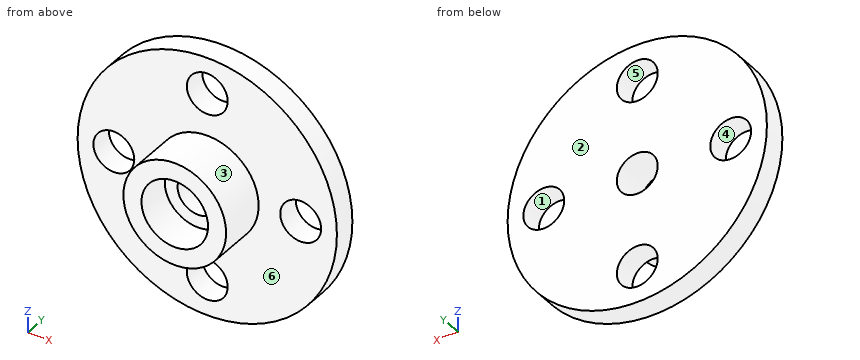
```python
from build123d import *

# Parameters (mm, degrees)
SKETCH1_R          = 11.1
EXTRUDE1_DEPTH     = 2
SKETCH2_R          = 1.75
CUT_EXTRUDE1_DEPTH = 3
SKETCH3_R          = 4.4
EXTRUDE2_DEPTH     = 4.2
SKETCH4_R          = 2.85
CUT_EXTRUDE2_DEPTH = 3
SKETCH5_R          = 1.75
CUT_EXTRUDE3_DEPTH = 4.2


with BuildPart() as part:
    # Sketch1 → Extrude1 (new body)
    with BuildSketch(Plane(origin=(0, 0, 0), x_dir=(1, 0, 0), z_dir=(0, 1, 0))):
        Circle(SKETCH1_R)
    extrude(amount=EXTRUDE1_DEPTH)

    # Sketch2 → Cut-Extrude1 (cut, through all)
    with BuildSketch(Plane(origin=(0, 2, 0), x_dir=(1, 0, 0), z_dir=(0, 1, 0))):
        with Locations((0, 8)):
            Circle(SKETCH2_R)
        with Locations((8, 0)):
            Circle(SKETCH2_R)
        with Locations((0, -8)):
            Circle(SKETCH2_R)
        with Locations((-8, 0)):
            Circle(SKETCH2_R)
    extrude(amount=-CUT_EXTRUDE1_DEPTH, mode=Mode.SUBTRACT)

    # Sketch3 → Extrude2 (add)
    with BuildSketch(Plane.XZ):
        Circle(SKETCH3_R)
    extrude(amount=EXTRUDE2_DEPTH)

    # Sketch4 → Cut-Extrude2 (cut)
    with BuildSketch(Plane.XZ.offset(4.2)):
        Circle(SKETCH4_R)
    extrude(amount=-CUT_EXTRUDE2_DEPTH, mode=Mode.SUBTRACT)

    # Sketch5 → Cut-Extrude3 (cut, through all)
    with BuildSketch(Plane.XZ.offset(1.2)):
        Circle(SKETCH5_R)
    extrude(amount=-CUT_EXTRUDE3_DEPTH, mode=Mode.SUBTRACT)


solid = part.part
```
Can you work these out from the model? Positions are in its coordinate system, mm. Face numbers are marked on the shaded views. A direction names the side the tool comes from. Coordinates: 2 decimals unless noted, no trailing zeros. Order: outer loops, then holes, each group sorted by start corner. A loop starts at its lowest first (then second) coordinate and runs counter-clockwise, first axis right, second up.
1. For the marked faces 5 and 6, which set-ups out of +Z, -Z, +X, -X, +Y, -Y let a thin tool reach every point of the face, with its end or its side?
2. If we section it at A-A (z = 0): Please give me the cut outline in (x, y).
3. If we section it at D-D (y = 0.5): Please give me the cut outline in (x, z).
4. Thinking about a two-plate mould opening in Z: for the marked faces 1, 2, 3 and 4, which applies, +Z half, -Z half, draft (parallel to the pull), parting line (faces both ways), or undercut?
5. If we section it at C-C (x = -8): Please give me the cut outline in (y, z), then the cut area to 3 significant figures.
6. If we section it at B-B (x = 0): Please give me the cut outline in (y, z), then the cut area to 3 significant figures.
7. I'm going to push a flat-ended pin straight in: pin 1 (4 mm diameter, centred on x = 0, z = 8, fed in from -Y). Where does the tip first touch, or does it pass through?
8. I need wall thicknesses on line 1 (Z direction, x = 0, y = 0.5); line 2 (Z direction, x = 0, y = -2.25); line 3 (X direction, y = 1.25, z = 8.25). Which ranges of each line are inside material? Lowest first, please.
Entries:
1. face 5: +Y, -Y
1. face 6: -Y
2. outline: (-11.1, 0) - (-9.75, 0) - (-9.75, 2) - (-11.1, 2) - close; (-6.25, 0) - (-4.4, 0) - (-4.4, -4.2) - (-2.85, -4.2) - (-2.85, -1.2) - (-1.75, -1.2) - (-1.75, 2) - (-6.25, 2) - close; (1.75, -1.2) - (2.85, -1.2) - (2.85, -4.2) - (4.4, -4.2) - (4.4, 0) - (6.25, 0) - (6.25, 2) - (1.75, 2) - close; (9.75, 0) - (11.1, 0) - (11.1, 2) - (9.75, 2) - close
3. outline: circle Ø22.2 at (0, 0); hole circle Ø3.5 at (-8, 0); hole circle Ø3.5 at (0, -8); hole circle Ø3.5 at (0, 0); hole circle Ø3.5 at (0, 8); hole circle Ø3.5 at (8, 0)
4. face 1: undercut
4. face 2: draft
4. face 3: parting line
4. face 4: undercut
5. outline: (0, -7.69) - (2, -7.69) - (2, -1.75) - (0, -1.75) - close; (0, 1.75) - (2, 1.75) - (2, 7.69) - (0, 7.69) - close
5. area: 23.8 mm2
6. outline: (-4.2, -4.4) - (0, -4.4) - (0, -6.25) - (2, -6.25) - (2, -1.75) - (-1.2, -1.75) - (-1.2, -2.85) - (-4.2, -2.85) - close; (-4.2, 2.85) - (-1.2, 2.85) - (-1.2, 1.75) - (2, 1.75) - (2, 6.25) - (0, 6.25) - (0, 4.4) - (-4.2, 4.4) - close; (0, -11.1) - (2, -11.1) - (2, -9.75) - (0, -9.75) - close; (0, 9.75) - (2, 9.75) - (2, 11.1) - (0, 11.1) - close
6. area: 39.1 mm2
7. pin 1: stops at y = 0
8. line 1: z = -11.1 to -9.75, -6.25 to -1.75, 1.75 to 6.25, 9.75 to 11.1
8. line 2: z = -4.4 to -2.85, 2.85 to 4.4
8. line 3: x = -7.43 to -1.73, 1.73 to 7.43
